```python
from build123d import *

# Parameters (mm, degrees)
SKETCH1_R           = 11
SKETCH1_R_2         = 2.5
SKETCH1_R_3         = 2.1
SKETCH1_R_4         = 1.5
BOSS_EXTRUDE1_DEPTH = 2.5
CUT_EXTRUDE1_DEPTH  = 84.254129027
SKETCH3_R           = 2
CUT_EXTRUDE2_DEPTH  = 84.254129027
FILLET1_R           = 0.4
FILLET2_R           = 2


with BuildPart() as part:
    # Sketch1 → Boss-Extrude1 (new, symmetric)
    with BuildSketch(Plane.XY):
        with BuildLine():
            Line((-30, -47.5), (-22.5, -47.5))
            Line((-22.5, -47.5), (-22.5, -46.8))
            ThreePointArc((-22.5, -46.8), (-23.8, -45.5), (-22.5, -44.2))
            Line((-22.5, -44.2), (-20.5, -44.2))
            ThreePointArc((-20.5, -44.2), (-19.2, -45.5), (-20.5, -46.8))
            Line((-20.5, -46.8), (-20.5, -47.5))
            Line((-20.5, -47.5), (20.5, -47.5))
            Line((20.5, -47.5), (20.5, -46.8))
            ThreePointArc((20.5, -46.8), (19.2, -45.5), (20.5, -44.2))
            Line((20.5, -44.2), (22.5, -44.2))
            ThreePointArc((22.5, -44.2), (23.8, -45.5), (22.5, -46.8))
            Line((22.5, -46.8), (22.5, -47.5))
            Line((22.5, -47.5), (30, -47.5))
            Line((30, -47.5), (30, 47.5))
            ThreePointArc((30, 47.5), (0, 77.5), (-30, 47.5))
            Line((-30, 47.5), (-30, -47.5))
        make_face()
        with Locations((0, 47.5)):
            Circle(SKETCH1_R, mode=Mode.SUBTRACT)
        with Locations((21.5, -35.5)):
            Circle(SKETCH1_R_2, mode=Mode.SUBTRACT)
        with Locations((-21.5, -35.5)):
            Circle(SKETCH1_R_2, mode=Mode.SUBTRACT)
        with Locations((0, 30)):
            Circle(SKETCH1_R_3, mode=Mode.SUBTRACT)
        with Locations((-17.5, 47.5)):
            Circle(SKETCH1_R_3, mode=Mode.SUBTRACT)
        with Locations((0, 65)):
            Circle(SKETCH1_R_3, mode=Mode.SUBTRACT)
        with Locations((17.5, 47.5)):
            Circle(SKETCH1_R_3, mode=Mode.SUBTRACT)
        with Locations((-27, 0.779569979)):
            Circle(SKETCH1_R_4, mode=Mode.SUBTRACT)
        with Locations((-1.65030964, 10.779569979)):
            Circle(SKETCH1_R_4, mode=Mode.SUBTRACT)
        with Locations((16, 2.529392469)):
            Circle(SKETCH1_R_4, mode=Mode.SUBTRACT)
        with Locations((-15, 2.529392469)):
            Circle(SKETCH1_R_4, mode=Mode.SUBTRACT)
        with BuildLine():
            Line((20.5, -28.1), (22.5, -28.1))
            ThreePointArc((22.5, -28.1), (23.9, -29.5), (22.5, -30.9))
            Line((22.5, -30.9), (20.5, -30.9))
            ThreePointArc((20.5, -30.9), (19.1, -29.5), (20.5, -28.1))
        make_face(mode=Mode.SUBTRACT)
        with BuildLine():
            Line((-20.5, -28.1), (-22.5, -28.1))
            ThreePointArc((-22.5, -28.1), (-23.9, -29.5), (-22.5, -30.9))
            Line((-22.5, -30.9), (-20.5, -30.9))
            ThreePointArc((-20.5, -30.9), (-19.1, -29.5), (-20.5, -28.1))
        make_face(mode=Mode.SUBTRACT)
    extrude(amount=BOSS_EXTRUDE1_DEPTH, both=True)

    # Sketch2 → Cut-Extrude1 (cut, through all)
    with BuildSketch(Plane(origin=(0, 0, -2.5), x_dir=(-1, 0, 0), z_dir=(0, 0, -1))):
        with BuildLine():
            Line((8.51843153, 11.388546871), (18.855050358, 15.150768448))
            ThreePointArc((18.855050358, 15.150768448), (20.349231552, 18.355050358), (17.144949642, 19.849231552))
            Line((17.144949642, 19.849231552), (6.808330813, 16.087009975))
            ThreePointArc((6.808330813, 16.087009975), (5.314149619, 12.882728065), (8.51843153, 11.388546871))
        make_face()
    extrude(amount=-CUT_EXTRUDE1_DEPTH, mode=Mode.SUBTRACT)

    # Sketch3 → Cut-Extrude2 (cut, through all)
    with BuildSketch(Plane.XY.offset(2.5)):
        with Locations((13, -17.5)):
            Circle(SKETCH3_R)
        with Locations((20, -17.5)):
            Circle(SKETCH3_R)
        with Locations((13, 22.5)):
            Circle(SKETCH3_R)
        with Locations((20, 22.5)):
            Circle(SKETCH3_R)
    extrude(amount=-CUT_EXTRUDE2_DEPTH, mode=Mode.SUBTRACT)

    # Fillet1
    # the kernel refuses this fillet: 0.4 mm, written as the material it takes off along each edge
    with BuildSketch(Plane(origin=(22.5, -47.5, -3.5), x_dir=(1, 0, 0), z_dir=(0, 0, 1))) as fillet1_piece_1:
        with BuildLine():
            CenterArc((FILLET1_R, FILLET1_R), FILLET1_R, 180, 90)
            Line((0, FILLET1_R), (0, 0))
            Line((0, 0), (FILLET1_R, 0))
        make_face()
    extrude(amount=7, mode=Mode.SUBTRACT)
    with BuildSketch(Plane(origin=(22.5, -46.8, -3.38067791), x_dir=(0, -1, 0), z_dir=(0, 0, 1))) as fillet1_piece_2:
        with BuildLine():
            CenterArc((0.352271164, 0.4), FILLET1_R, 193.608960631, 76.391039369)
            ThreePointArc((-0.036498522, 0.305882353), (-0.00915688, 0.154026098), (0, 0))
            Line((0, 0), (0.352271164, 0))
        make_face()
    extrude(amount=6.761355821, mode=Mode.SUBTRACT)
    with BuildSketch(Plane(origin=(20.5, -47.5, -3.5), x_dir=(-1, 0, 0), z_dir=(0, 0, 1)), Plane(origin=(-20.5, -47.5, -3.5), x_dir=(0, 1, 0), z_dir=(0, 0, 1)), Plane(origin=(-22.5, -47.5, -3.5), x_dir=(-1, 0, 0), z_dir=(0, 0, 1))) as fillet1_piece_3:
        with BuildLine():
            CenterArc((FILLET1_R, -FILLET1_R), FILLET1_R, 90, 90)
            Line((0, -FILLET1_R), (0, 0))
            Line((0, 0), (FILLET1_R, 0))
        make_face()
    extrude(amount=7, mode=Mode.SUBTRACT)
    with BuildSketch(Plane(origin=(20.5, -46.8, -3.38067791), x_dir=(-0.9929562463238142, 0.11848161412860948, 0), z_dir=(0, 0, 1))) as fillet1_piece_4:
        with BuildLine():
            CenterArc((0.355444842, 0.397182499), FILLET1_R, 186.804480315, 76.391039369)
            Line((-0.041737656, 0.349789853), (0, 0))
            ThreePointArc((0, 0), (0.154026098, 0.00915688), (0.308052197, 0))
        make_face()
    extrude(amount=6.761355821, mode=Mode.SUBTRACT)
    with BuildSketch(Plane(origin=(-20.5, -46.8, -3.38067791), x_dir=(0.9929562463238113, 0.11848161412863496, 0), z_dir=(0, 0, 1))) as fillet1_piece_5:
        with BuildLine():
            CenterArc((0.355444842, -0.397182499), FILLET1_R, 96.804480315, 76.391039369)
            Line((-0.041737656, -0.349789853), (0, 0))
            ThreePointArc((0, 0), (0.154026098, -0.00915688), (0.308052197, 0))
        make_face()
    extrude(amount=6.761355821, mode=Mode.SUBTRACT)
    with BuildSketch(Plane(origin=(-22.5, -46.8, -3.38067791), x_dir=(0, -1, 0), z_dir=(0, 0, 1))) as fillet1_piece_6:
        with BuildLine():
            CenterArc((0.352271164, -0.4), FILLET1_R, 90, 76.391039369)
            ThreePointArc((-0.036498522, -0.305882353), (-0.00915688, -0.154026098), (0, 0))
            Line((0, 0), (0.352271164, 0))
        make_face()
    extrude(amount=6.761355821, mode=Mode.SUBTRACT)

    # Fillet2
    fillet2_edges = [part.edges().sort_by_distance(p)[0] for p in [
        (30, -47.5, 0),
        (-30, -47.5, 0),
    ]]
    fillet(fillet2_edges, radius=FILLET2_R)


solid = part.part
```
The model under review builds one solid part; all positions refer to its coordinate system, in mm. A direction names the side the tool comes from. Round coordinates to 2 decimals unless told otherwise and drop trailing zeros. Write each loop counter-clockwise with the first axis right and the second up, starting at its lowest first coordinate (ties: lowest second). Pieces come first, ordered by that corner, then holes. Notation, with made-up numbers: (22, 1) - (45, 1) arc R14 cw to (45, 28) - close; hole circle Ø2 at (35, 47.25). An arc over 180 degrees is marked (long way). Answer as CSV lines item,"result". Start each with the question number.
(1) For pin 1 Ø1.6 at (x, z) = (21.5, 0.5) entering from -Y; pin 2 Ø1 at (x, z) = (21.5, 0.5) entering from +Y; pin 3 Ø1.6 at (x, z) = (-22, -1) entering from -Y, all flat-tipped, find the tip position at first contact; note any pin that passes through.
(2) We need section C-C on y = 52.5. State the section outline as (x, z) points, plus the area to 3 significant figures.
(3) For faces 3 (the cylindrical face through (23.9, -29.5, 0)), 4 (the flat face through (0, -47.5, 0)), list the 3-axis set-ups (+Z, -Z, +X, -X, +Y, -Y) from which the entire face can be reached by the end or side of a thin tool; tool diameter is ignored.
(4) Draft analysis for pull direction X (two halves, no side actions). For faces 1 (the cylindrical face through (-1.666, 63.722, -0.035)), 2 (the flat face through (25, -47.5, 0)), state which applies: pulls with the +X half, pulls with the -X half, needs draft (parallel to the pull), parting line crosses it, or undercut.
(5) We need section B-B on x = 13. State the section outline as (y, z) points.
(6) We need section D-D on y = 17.5. State the section outline as (x, z) points, plus the area to 3 significant figures.
(7) To check wall thickness, follow line 1 (Y direction, x = 0, z = 0.9); line 2 (Y direction, x = -17.5, z = 1.1); line 3 (Y direction, x = -6.5, z = -2.15). State the ranges of each line that lie inside material, in increasing order.
(8) We need section A-A on y = -17.5. State the section outline as (x, z) points.
Worked answers:
1,pin 1,"y = -44.2"
1,pin 2,"y = 68.92"
1,pin 3,"y = -47.49"
2,outline,"(-29.58, -2.5) - (-9.8, -2.5) - (-9.8, 2.5) - (-29.58, 2.5) - close; (9.8, -2.5) - (29.58, -2.5) - (29.58, 2.5) - (9.8, 2.5) - close"
2,area,"198 mm²"
3,face 3,"+Z, -Z"
3,face 4,"+Z, -Z, +X, -X, -Y"
4,face 1,"undercut"
4,face 2,"needs draft"
5,outline,"(-47.5, -2.5) - (-19.5, -2.5) - (-19.5, 2.5) - (-47.5, 2.5) - close; (-15.5, -2.5) - (20.5, -2.5) - (20.5, 2.5) - (-15.5, 2.5) - close; (24.5, -2.5) - (74.54, -2.5) - (74.54, 2.5) - (24.5, 2.5) - close"
6,outline,"(-30, -2.5) - (-20.5, -2.5) - (-20.5, 2.5) - (-30, 2.5) - close; (-10.69, -2.5) - (30, -2.5) - (30, 2.5) - (-10.69, 2.5) - close"
6,area,"251 mm²"
7,line 1,"-47.5 to 27.9, 32.1 to 36.5, 58.5 to 62.9, 67.1 to 77.5"
7,line 2,"-47.5 to 14.66, 19.95 to 45.4, 49.6 to 71.87"
7,line 3,"-47.5 to 11.52, 15.95 to 38.63, 56.37 to 76.79"
8,outline,"(-30, -2.5) - (11, -2.5) - (11, 2.5) - (-30, 2.5) - close; (15, -2.5) - (18, -2.5) - (18, 2.5) - (15, 2.5) - close; (22, -2.5) - (30, -2.5) - (30, 2.5) - (22, 2.5) - close"
